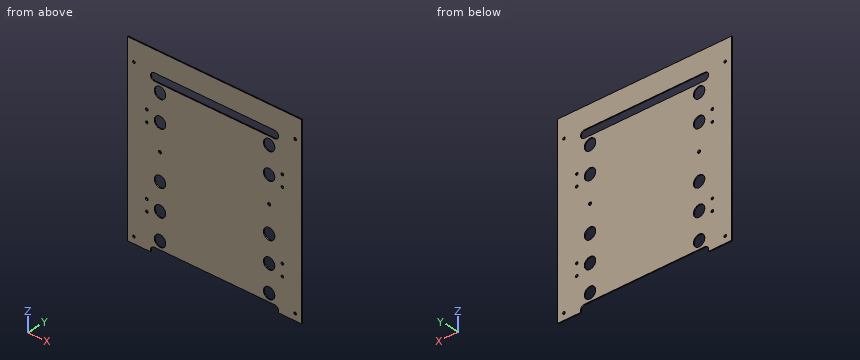
from build123d import *

# Parameters (mm, degrees)
SKETCH1_R           = 2.15265
SKETCH1_R_2         = 9.525
SKETCH1_R_3         = 2.4892
BOSS_EXTRUDE1_DEPTH = 1.5875


with BuildPart() as part:
    # Sketch1 → Boss-Extrude1 (new body)
    with BuildSketch(Plane(origin=(0, 0, 0), x_dir=(1, 0, 0), z_dir=(0, 1, 0))):
        with BuildLine():
            Line((-107.315, 152.4), (-146.05, 152.4))
            Line((-146.05, 152.4), (-146.05, -152.4))
            Line((-146.05, -152.4), (146.05, -152.4))
            Line((146.05, -152.4), (146.05, 152.4))
            Line((146.05, 152.4), (107.315, 152.4))
            Line((107.315, 152.4), (107.315, 149.225))
            ThreePointArc((107.315, 149.225), (105.455128061, 144.734871939), (100.965, 142.875))
            Line((100.965, 142.875), (-100.965, 142.875))
            ThreePointArc((-100.965, 142.875), (-105.455128061, 144.734871939), (-107.315, 149.225))
            Line((-107.315, 149.225), (-107.315, 152.4))
        make_face()
        with Locations(Location((-135.128, -118.872, 0), (0, 0, 270))):
            Circle(SKETCH1_R, mode=Mode.SUBTRACT)
        with Locations(Location((-91.44, -91.44, 0), (0, 0, 270))):
            Circle(SKETCH1_R_2, mode=Mode.SUBTRACT)
        with Locations(Location((-113.665, -57.15, 0), (0, 0, 270))):
            Circle(SKETCH1_R, mode=Mode.SUBTRACT)
        with Locations(Location((-113.665, -38.1, 0), (0, 0, 270))):
            Circle(SKETCH1_R, mode=Mode.SUBTRACT)
        with Locations(Location((-91.44, -47.244, 0), (0, 0, 270))):
            Circle(SKETCH1_R_2, mode=Mode.SUBTRACT)
        with Locations(Location((-91.44, -3.048, 0), (0, 0, 270))):
            Circle(SKETCH1_R_3, mode=Mode.SUBTRACT)
        with BuildLine():
            ThreePointArc((-100.965, -117.475), (-107.315, -111.125), (-100.965, -104.775))
            Line((-100.965, -104.775), (100.965, -104.775))
            ThreePointArc((100.965, -104.775), (107.315, -111.125), (100.965, -117.475))
            Line((100.965, -117.475), (-100.965, -117.475))
        make_face(mode=Mode.SUBTRACT)
        with Locations(Location((135.128, -118.872, 0), (0, 0, 270))):
            Circle(SKETCH1_R, mode=Mode.SUBTRACT)
        with Locations(Location((91.44, -91.44, 0), (0, 0, 270))):
            Circle(SKETCH1_R_2, mode=Mode.SUBTRACT)
        with Locations(Location((91.44, -47.244, 0), (0, 0, 270))):
            Circle(SKETCH1_R_2, mode=Mode.SUBTRACT)
        with Locations(Location((113.665, -57.15, 0), (0, 0, 270))):
            Circle(SKETCH1_R, mode=Mode.SUBTRACT)
        with Locations(Location((113.665, -38.1, 0), (0, 0, 270))):
            Circle(SKETCH1_R, mode=Mode.SUBTRACT)
        with Locations(Location((91.44, -3.048, 0), (0, 0, 270))):
            Circle(SKETCH1_R_3, mode=Mode.SUBTRACT)
        with Locations(Location((-113.665, 76.2, 0), (0, 0, 270))):
            Circle(SKETCH1_R, mode=Mode.SUBTRACT)
        with Locations(Location((-91.44, 41.148, 0), (0, 0, 270))):
            Circle(SKETCH1_R_2, mode=Mode.SUBTRACT)
        with Locations(Location((-113.665, 95.25, 0), (0, 0, 270))):
            Circle(SKETCH1_R, mode=Mode.SUBTRACT)
        with Locations(Location((-91.44, 85.344, 0), (0, 0, 270))):
            Circle(SKETCH1_R_2, mode=Mode.SUBTRACT)
        with Locations(Location((-135.128, 141.478, 0), (0, 0, 270))):
            Circle(SKETCH1_R, mode=Mode.SUBTRACT)
        with Locations(Location((-91.44, 129.54, 0), (0, 0, 270))):
            Circle(SKETCH1_R_2, mode=Mode.SUBTRACT)
        with Locations(Location((91.44, 41.148, 0), (0, 0, 270))):
            Circle(SKETCH1_R_2, mode=Mode.SUBTRACT)
        with Locations(Location((113.665, 76.2, 0), (0, 0, 270))):
            Circle(SKETCH1_R, mode=Mode.SUBTRACT)
        with Locations(Location((91.44, 85.344, 0), (0, 0, 270))):
            Circle(SKETCH1_R_2, mode=Mode.SUBTRACT)
        with Locations(Location((113.665, 95.25, 0), (0, 0, 270))):
            Circle(SKETCH1_R, mode=Mode.SUBTRACT)
        with Locations(Location((91.44, 129.54, 0), (0, 0, 270))):
            Circle(SKETCH1_R_2, mode=Mode.SUBTRACT)
        with Locations(Location((135.128, 141.478, 0), (0, 0, 270))):
            Circle(SKETCH1_R, mode=Mode.SUBTRACT)
    extrude(amount=BOSS_EXTRUDE1_DEPTH)


solid = part.part
Work out the finished part from the listing and answer in its coordinate system (mm). Coordinates: 2 decimals unless noted, no trailing zeros. Write each loop counter-clockwise with the first axis right and the second up, starting at its lowest first coordinate (ties: lowest second). Pieces come first, ordered by that corner, then holes. Notation, with made-up numbers: M 39,49.5 L 93,49.5 A21 ccw 93,53.5 Z; hole C -37,22.25 d7. An arc over 180 degrees is marked long. Use one line per item in the form item = value. Start each with the question number.
1. The part is cut by section B-B (z = 91.44). Give the number of separate pieces and of enclosed holes in the cut face, plus the area to 3 significant figures.
2. Straight lines are drawn through the part: probe 1 along X at (y, z) = (0.7, 91.44) (3 decimals); probe 2 along Z at (x, y) = (-67.5, 0.65) (3 decimals); probe 3 along X at (y, z) = (0.6, -42.5). For each, find the intervals that lie inside material, in ascending order. Write a range as from..to.
3. This flat-tipped pin is pushed along its axis until it touches: P1, Ø2.5, axis at x = 113.665, z = -76.2, coming from the -Y side. Where does it stop, or does it pass through?
4. The part is cut by section A-A (x = -5). Give the vertices of the cut face in (y, z) (1 decimal), plus the area to 3 significant figures.
Evaluation:
q1.separate_pieces = 3
q1.enclosed_holes = 0
q1.area = 403 mm^2
q2.probe_1 = -146.05..-100.965, -81.915..81.915, 100.965..146.05
q2.probe_2 = -142.875..104.775, 117.475..152.4
q2.probe_3 = -146.05..-100.87, -82.01..82.01, 100.87..146.05
q3.P1 = through
q4.outline = M 0,-142.9 L 1.6,-142.9 L 1.6,104.8 L 0,104.8 Z; M 0,117.5 L 1.6,117.5 L 1.6,152.4 L 0,152.4 Z
q4.area = 449 mm^2
